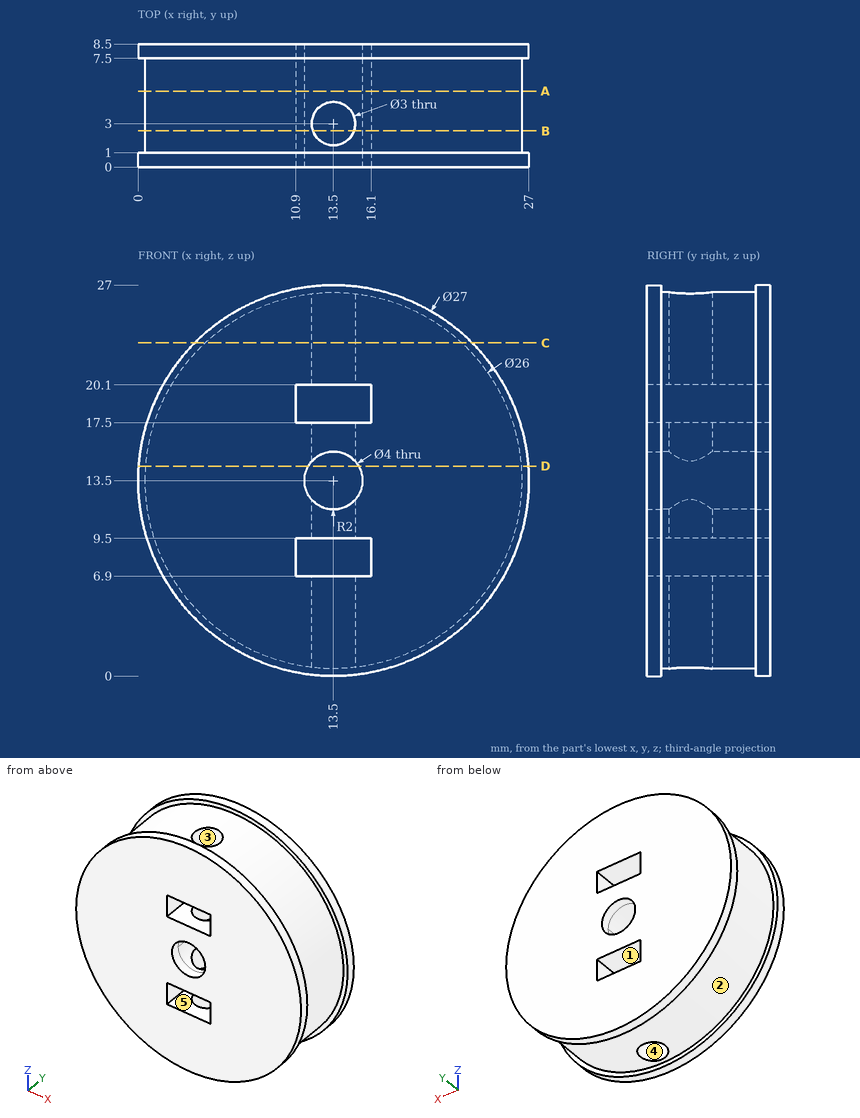
Could you check a few things on this drawing? It's one solid part, dimensions in mm from its lowest x, y, z. A direction names the side the tool comes from. Coordinates: 2 decimals unless noted, no trailing zeros. Loops run counter-clockwise (first coordinate to the right, second up) from the corner with the lowest first, then second, coordinate; pieces in that order, holes last. Notation, with made-up numbers: (75, 47.5) - (95, 47.5) arc R13 ccw to (95, 55.5) - close; hole circle Ø6 at (-28.75, -17). An arc over 180 degrees is marked (long way). Answer as a JSON object with one key per item and string values. Group by question number.
Item 1: For pin 1 (8 mm diameter, centred on x = 9.5, z = 8.5, fed in from -Y); pin 2 (2.5 mm diameter, centred on x = 13.5, y = 3, fed in from +Z); pin 3 (3 mm diameter, centred on y = 4.5, z = 19, fed in from -X); pin 4 (0.8 mm diameter, centred on y = 4.5, z = 8, fed in from -X), each with a flat end and sliding along its axis, tell me the tip position at first contact or that it passes through.
Item 2: If we mould it in two halves opening along Z, with no side actions, what happens to the marked faces 1, 2 and 3? For each: released by +Z, released by -Z, zero draft, split by the parting line, or undercut.
Item 3: If we section it at A-A (y = 5.25): List the corners of the cut face in (x, z) for me, plus the area to 3 significant figures.
Item 4: If we section it at C-C (z = 23): List the corners of the cut face in (x, y) for me.
Item 5: If we section it at B-B (y = 2.5): List the corners of the cut face in (x, z) for me.
Item 6: If I drill on L1, parallel to Y at x = 13.5, z = 22; L2, parallel to Y at x = 20.5, z = 24.5; L3, parallel to X at y = 3, z = 13.75, over which ranges is the centre line in solid material (lowest first)? Write a range as from..to.
Item 7: On a 3-axis mill with a long thin cutter (end or side, diameter ignored), from which of +Z, -Z, +X, -X, +Y, -Y can I reach the whole of each face in a straight line? I mean the marked faces 4 and 5. Say none if no direction works.
Item 8: If we section it at D-D (z = 14.5): List the corners of the cut face in (x, y) for me.
Returned:
{
 "1": {"pin 1": "stops at y = 0", "pin 2": "passes through", "pin 3": "stops at x = 1.13", "pin 4": "stops at x = 1.54"},
 "2": {"face 1": "undercut", "face 2": "split by the parting line", "face 3": "zero draft"},
 "3": {"outline": "circle Ø26 at (13.5, 13.5); hole (10.9, 6.9) - (16.1, 6.9) - (16.1, 9.5) - (10.9, 9.5) - close; hole (10.9, 17.5) - (16.1, 17.5) - (16.1, 20.1) - (10.9, 20.1) - close; hole circle Ø4 at (13.5, 13.5)", "area": "491 mm²"},
 "4": {"outline": "(3.91, 0) - (23.09, 0) - (23.09, 1) - (22.37, 1) - (22.37, 7.5) - (23.09, 7.5) - (23.09, 8.5) - (3.91, 8.5) - (3.91, 7.5) - (4.63, 7.5) - (4.63, 1) - (3.91, 1) - close; hole circle Ø3 at (13.5, 3)"},
 "5": {"outline": "(10.9, 6.9) - (10.9, 9.5) - (12.09, 9.5) - (12.09, 12.09) arc R2 cw to (12.09, 14.91) - (12.09, 17.5) - (10.9, 17.5) - (10.9, 20.1) - (12.09, 20.1) - (12.09, 26.42) arc R13 ccw to (12.09, 0.58) - (12.09, 6.9) - close; (14.91, 0.58) arc R13 ccw to (14.91, 26.42) - (14.91, 20.1) - (16.1, 20.1) - (16.1, 17.5) - (14.91, 17.5) - (14.91, 14.91) arc R2 cw to (14.91, 12.09) - (14.91, 9.5) - (16.1, 9.5) - (16.1, 6.9) - (14.91, 6.9) - close"},
 "6": {"L1": "y = 0..1.5, 4.5..8.5", "L2": "y = 0..1, 7.5..8.5", "L3": "x = 0.5..11.52, 15.48..26.5"},
 "7": {"face 4": "+Z, -Z", "face 5": "+Y, -Y"},
 "8": {"outline": "(0.04, 0) - (11.77, 0) - (11.77, 8.5) - (0.04, 8.5) - (0.04, 7.5) - (0.54, 7.5) - (0.54, 1) - (0.04, 1) - close; (15.23, 0) - (26.96, 0) - (26.96, 1) - (26.46, 1) - (26.46, 7.5) - (26.96, 7.5) - (26.96, 8.5) - (15.23, 8.5) - close"}
}
